from build123d import *

# Parameters (mm, degrees)
ESQUISSE1_R                = 6
ESQUISSE1_R_2              = 5
BOSS_EXTRU_1_DEPTH         = 20
ESQUISSE2_R                = 6
ESQUISSE2_R_2              = 4.5
BOSS_EXTRU_2_DEPTH         = 1
ESQUISSE3_R                = 7.5
ESQUISSE3_R_2              = 5
BOSS_EXTRU_3_DEPTH         = 7
ESQUISSE4_R                = 8
ESQUISSE4_R_2              = 5
BOSS_EXTRU_4_DEPTH         = 2
ESQUISSE7_R                = 6
ESQUISSE7_R_2              = 5
BOSS_EXTRU_7_DEPTH         = 11
ESQUISSE8_R                = 8
ESQUISSE8_R_2              = 5
BOSS_EXTRU_8_DEPTH         = 2
D_GAGEMENT_M41_D           = 4.5
D_GAGEMENT_M41_ON_FACE_2_D = 4.5
ESQUISSE15_R               = 7.5
ESQUISSE15_R_2             = 5
BOSS_EXTRU_9_DEPTH         = 7
ESQUISSE16_R               = 5.5
ESQUISSE16_R_2             = 5
BOSS_EXTRU_10_DEPTH        = 5
ESQUISSE17_W               = 20
ESQUISSE17_H               = 2
ESQUISSE17_W_2             = 2
ESQUISSE17_H_2             = 20
ENL_V_MAT_EXTRU_1_DEPTH    = 5


with BuildPart() as part:
    # Esquisse1 → Boss.-Extru.1 (new body)
    with BuildSketch(Plane.XY):
        Circle(ESQUISSE1_R)
        Circle(ESQUISSE1_R_2, mode=Mode.SUBTRACT)
    extrude(amount=BOSS_EXTRU_1_DEPTH)

    # Esquisse2 → Boss.-Extru.2 (add)
    with BuildSketch(Plane(origin=(0, 0, 0), x_dir=(-1, 0, 0), z_dir=(0, 0, -1))):
        Circle(ESQUISSE2_R)
        Circle(ESQUISSE2_R_2, mode=Mode.SUBTRACT)
    extrude(amount=-BOSS_EXTRU_2_DEPTH)

    # Esquisse3 → Boss.-Extru.3 (add)
    with BuildSketch(Plane.XY.offset(20)):
        Circle(ESQUISSE3_R)
        Circle(ESQUISSE3_R_2, mode=Mode.SUBTRACT)
    extrude(amount=BOSS_EXTRU_3_DEPTH)

    # Esquisse4 → Boss.-Extru.4 (add)
    with BuildSketch(Plane.XY.offset(27)):
        Circle(ESQUISSE4_R)
        Circle(ESQUISSE4_R_2, mode=Mode.SUBTRACT)
    extrude(amount=BOSS_EXTRU_4_DEPTH)

    # Esquisse7 → Boss.-Extru.7 (add)
    with BuildSketch(Plane.XY.offset(29)):
        Circle(ESQUISSE7_R)
        Circle(ESQUISSE7_R_2, mode=Mode.SUBTRACT)
    extrude(amount=BOSS_EXTRU_7_DEPTH)

    # Esquisse8 → Boss.-Extru.8 (add)
    with BuildSketch(Plane.XY.offset(40)):
        Circle(ESQUISSE8_R)
        Circle(ESQUISSE8_R_2, mode=Mode.SUBTRACT)
    extrude(amount=BOSS_EXTRU_8_DEPTH)

    # Dégagement M41 (through all)
    with Locations(Plane(origin=(6, 0, 4), x_dir=(0, 1, 0), z_dir=(1, 0, 0))):
        with Locations((0, 0)):
            Hole(D_GAGEMENT_M41_D / 2)

    # Dégagement M41 on face 2 (through all)
    with Locations(Plane(origin=(0, 6, 4), x_dir=(0, 0, 1), z_dir=(0, 1, 0))):
        with Locations((0, 0)):
            Hole(D_GAGEMENT_M41_ON_FACE_2_D / 2)

    # Esquisse15 → Boss.-Extru.9 (add)
    with BuildSketch(Plane.XY.offset(42)):
        Circle(ESQUISSE15_R)
        Circle(ESQUISSE15_R_2, mode=Mode.SUBTRACT)
    extrude(amount=BOSS_EXTRU_9_DEPTH)

    # Esquisse16 → Boss.-Extru.10 (add)
    with BuildSketch(Plane.XY.offset(49)):
        Circle(ESQUISSE16_R)
        Circle(ESQUISSE16_R_2, mode=Mode.SUBTRACT)
    extrude(amount=BOSS_EXTRU_10_DEPTH)

    # Esquisse17 → Enlèv. mat.-Extru.1 (cut)
    with BuildSketch(Plane.XY.offset(54)):
        Rectangle(ESQUISSE17_W, ESQUISSE17_H)
        Rectangle(ESQUISSE17_W_2, ESQUISSE17_H_2)
    extrude(amount=-ENL_V_MAT_EXTRU_1_DEPTH, mode=Mode.SUBTRACT)


solid = part.part
CAD build for the part. Positions are in the model's coordinates, mm. A direction names the side the tool comes from. Round coordinates to 2 decimals unless told otherwise and drop trailing zeros. Write each loop counter-clockwise with the first axis right and the second up, starting at its lowest first coordinate (ties: lowest second). Pieces come first, ordered by that corner, then holes. Notation, with made-up numbers: M 27.25,21.5 L 48.25,21.5 A33 ccw 48.25,49.5 Z; hole C -16,69 d5. An arc over 180 degrees is marked long. Put each result on its own line as item: value. Start each with the question number.
1) Pin check, flat tips, straight feed: pin 1 Ø6 at (y, z) = (0, 4) entering from -X; pin 2 Ø3 at (x, y) = (0.5, 1.5) entering from +Z (3 decimals); pin 3 Ø8 at (x, y) = (0.5, 1.5) entering from +Z; pin 4 Ø3 at (x, z) = (-5, 22) entering from +Y. Stop position of each tip, or through.
2) 3-axis set-ups, long thin cutter, end or side, ignore diameter. For faces 1 (the cylindrical face through (2.307, -4.436, 27.129)), 2 (the cylindrical face through (5.54, -2.3, 9.86)), 3 (the cylindrical face through (-6, 0, 34)): which of +Z, -Z, +X, -X, +Y, -Y reach the whole face in a straight line?
3) Saw through at A-A, the plane z = 18. Write the cut outline in (x, y).
4) Drill centre lines: probe 1 along Z at (x, y) = (0, 5.6); probe 2 along Y at (x, z) = (0, 0.25); probe 3 along Z at (x, y) = (4, -6.5). Where is each one in solid material? Low to high. Write a range as [from, to].
5) Saw through at B-B, the plane z = 4. Write the cut outline in (x, y), and give its area (3 significant figures).
6) Saw through at C-C, the plane x = 0. Count the separate pieces of the cut face and the enclosed holes in it, and give its area (3 significant figures).
7) Pull direction Y, two halves, no side cores. Call faces 4 (the cylindrical face through (0.59, 4.46, 0.49)), 5 (the cylindrical face through (3.86, -3.92, 51.46)), 6 (the flat face through (-3.7, 3.7, 54)): pulls with the +Y half, pulls with the -Y half, needs draft (parallel to the pull), parting line crosses it, or undercut.
Resolved:
1. pin 1: x = -6
1. pin 2: through
1. pin 3: z = 54
1. pin 4: y = 6.63
2. face 1: +Z
2. face 2: -Z
2. face 3: none
3. outline: C 0,0 d12; hole C 0,0 d10
4. probe 1: [0, 1.75], [6.25, 49]
4. probe 2: [-6, -4.5], [4.5, 6]
4. probe 3: [27, 29], [40, 42]
5. outline: M -5.56,-2.25 A6 ccw -2.25,-5.56 L -2.25,-4.47 A5 cw -4.47,-2.25 Z; M -5.56,2.25 L -4.47,2.25 A5 cw -2.25,4.47 L -2.25,5.56 A6 ccw Z; M 2.25,-5.56 A6 ccw 5.56,-2.25 L 4.47,-2.25 A5 cw 2.25,-4.47 Z; M 2.25,4.47 A5 cw 4.47,2.25 L 5.56,2.25 A6 ccw 2.25,5.56 Z
5. area: 16.0 mm²
6. separate pieces: 4
6. enclosed holes: 0
6. area: 148 mm²
7. face 4: undercut
7. face 5: pulls with the -Y half
7. face 6: needs draft
